The model under review builds one solid part; all positions refer to its coordinate system, in mm. A direction names the side the tool comes from. Coordinates: 2 decimals unless noted, no trailing zeros. Order: outer loops, then holes, each group sorted by start corner. A loop starts at its lowest first (then second) coordinate and runs counter-clockwise, first axis right, second up. Notation, with made-up numbers: (58, 84.5) -> (82, 84.5) arc R8 ccw to (82, 89.5) -> close; hole circle Ø1 at (79.25, -4.5). An arc over 180 degrees is marked (long way). Use one line per item in the form item = value.
from build123d import *

# Parameters (mm, degrees)
EXTRUDE_2_DEPTH     = 150
CUT_EXTRUDE_2_DEPTH = 180.51323071


with BuildPart() as part:
    # 草图3 → 凸台-拉伸2 (new body)
    with BuildSketch(Plane.XY):
        Polygon((0, 0), (0, 10), (17, 10), (17, 58), (5, 70), (5, 85), (13, 85), (13, 73), (37, 73), (37, 85), (45, 85), (45, 70), (33, 58), (33, 10), (50, 10), (50, 0), align=None)
    extrude(amount=EXTRUDE_2_DEPTH)

    # 草图4 → 切除-拉伸2 (cut, through all)
    with BuildSketch(Plane(origin=(50, 0, 0), x_dir=(0, 0, -1), z_dir=(1, 0, 0))):
        Polygon((-135, 85), (-135, 20), (-125, 10), (-25, 10), (-15, 20), (-15, 85), align=None)
    extrude(amount=-CUT_EXTRUDE_2_DEPTH, mode=Mode.SUBTRACT)


solid = part.part
Item 1: We need section B-B (x = 41). Write out the cut boundary in (y, z).
Results found:
outline = (0, 0) -> (10, 0) -> (10, 150) -> (0, 150) -> close; (66, 0) -> (85, 0) -> (85, 15) -> (66, 15) -> close; (66, 135) -> (85, 135) -> (85, 150) -> (66, 150) -> close
Item 2: Clearance check with flat-ended pins moving along their axes: pin 1 (4.5 mm diameter, centred on y = 77.5, z = 140, fed in from -X); pin 2 (12 mm diameter, centred on x = 27, z = 6, fed in from +Y); pin 3 (4 mm diameter, centred on x = 6, z = 37.5, fed in from +Y). State where each tip first meets the part, or that it passes through.
Results found:
pin_1 = 5
pin_2 = 73
pin_3 = 10
Item 3: We need section C-C (y = 78). Write out the cut boundary in (x, z), plus the area to 3 significant figures.
Results found:
outline = (5, 0) -> (13, 0) -> (13, 15) -> (5, 15) -> close; (5, 135) -> (13, 135) -> (13, 150) -> (5, 150) -> close; (37, 0) -> (45, 0) -> (45, 15) -> (37, 15) -> close; (37, 135) -> (45, 135) -> (45, 150) -> (37, 150) -> close
area = 480 mm²
Item 4: We need section A-A (y = 50). Write out the cut boundary in (x, z), plus the area to 3 significant figures.
Results found:
outline = (17, 0) -> (33, 0) -> (33, 15) -> (17, 15) -> close; (17, 135) -> (33, 135) -> (33, 150) -> (17, 150) -> close
area = 480 mm²
Item 5: To check wall thickness, follow L1, parallel to Z at x = 21, y = 23; L2, parallel to Y at x = 19.5, z = 124; L3, parallel to Y at x = 38, z = 14.5. State the ranges of each line that lie inside material, in increasing order. Write a range as from..to.
Results found:
L1 = 0..15, 135..150
L2 = 0..10
L3 = 0..10, 63..85
Item 6: Draft analysis for pull direction Y (two halves, no side actions). For faces 1 (the face through (25, 73, 7)), 2 (the face through (13, 79, 142)), 3 (the face through (33, 34, 143)), state which applies: released by +Y, released by -Y, zero draft, split by the parting line, or undercut.
Results found:
face_1 = released by +Y
face_2 = zero draft
face_3 = undercut
Item 7: Tool access review of faces 4 (the face through (17, 34, 7)), 5 (the face through (25, 15, 20)), 6 (the face through (45, 78, 142)), 7 (the face through (39, 64, 142)), 8 (the face through (13, 79, 7)): name each direction out of +Z, -Z, +X, -X, +Y, -Y from which nothing blocks a thin tool from reaching the whole face with its end or side.
Results found:
face_4 = +Z, -Z, -X
face_5 = +X, -X, +Y
face_6 = +Z, -Z, +X, +Y
face_7 = +Z, -Z, +X
face_8 = +Z, -Z, +Y
Item 8: We need section D-D (z = 137). Write out the cut boundary in (x, y).
Results found:
outline = (0, 0) -> (50, 0) -> (50, 10) -> (33, 10) -> (33, 58) -> (45, 70) -> (45, 85) -> (37, 85) -> (37, 73) -> (13, 73) -> (13, 85) -> (5, 85) -> (5, 70) -> (17, 58) -> (17, 10) -> (0, 10) -> close
